Read the model definition and answer for the solid it produces. Units are mm, in the model's axes. A direction names the side the tool comes from. Give positions to 0.01 mm unless a question says otherwise; leave off trailing zeros. Order: outer loops, then holes, each group sorted by start corner. A loop starts at its lowest first (then second) coordinate and runs counter-clockwise, first axis right, second up. Notation, with made-up numbers: (49.25, 45) - (72.25, 45) arc R15 cw to (72.25, 69) - close; hole circle Ø3 at (52.25, 60). An arc over 180 degrees is marked (long way). Use a Markdown table: item, result. Add a question column.
1. Flat-ended cylindrical pins translate along their axes: P1, Ø5, axis at y = -18.5, z = 10, coming from the -X side; P2, Ø12, axis at y = -17.5, z = 13, coming from the -X side; P3, Ø8, axis at x = 19, z = 3, coming from the -Y side. Find the tip coordinate at first contact, or state that the pin passes through.
2. A cutting plane is placed at B-B on x = 0. Determine the outline of the cut face in (y, z).
3. For a pull along Y with two mould halves and no side action, classify faces 1 (the flat face through (14, -14, 0)), 2 (the cylindrical face through (-20.514, 13.631, 9.86)), 3 (the cylindrical face through (-6.94, -31.24, 9.86)) as released by +Y, released by -Y, zero draft, split by the parting line, or undercut.
4. Which of the six approach directions +Z, -Z, +X, -X, +Y, -Y give full straight-line access (tool end or side, diameter ignored) to faces 4 (the flat face through (14, -14, 20)), 5 (the flat face through (-19, -15, 10))?
5. Consider L1, parallel to Y at x = 0, z = 15; L2, parallel to Y at x = 23.5, z = 17.25; L3, parallel to X at y = -13.5, z = 2.75. Determine where each line is inside the solid, lowest interval first.
6. A cutting plane is placed at D-D on y = 13. Determine the outline of the cut face in (x, z).
7. A cutting plane is placed at C-C on z = 7.25. Determine the outline of the cut face in (x, y), and give its area (3 significant figures).
8. A cutting plane is placed at A-A on y = 0. Determine the outline of the cut face in (x, z).
```python
from build123d import *

# Parameters (mm, degrees)
SKETCH_R     = 32
SKETCH_R_2   = 2.1
SKETCH_R_3   = 3
SKETCH_R_4   = 17.5
PAD_DEPTH    = 20
SKETCH001_R  = 5.5
POCKET_DEPTH = 10


with BuildPart() as part:
    # Sketch → Pad (new body)
    with BuildSketch(Plane.XY):
        Circle(SKETCH_R)
        with Locations((0, -26)):
            Circle(SKETCH_R_2, mode=Mode.SUBTRACT)
        with Locations((-22.51666, 13)):
            Circle(SKETCH_R_2, mode=Mode.SUBTRACT)
        with Locations((22.51666, 13)):
            Circle(SKETCH_R_2, mode=Mode.SUBTRACT)
        with Locations((0, 25)):
            Circle(SKETCH_R_3, mode=Mode.SUBTRACT)
        with Locations((-21.650635, -12.5)):
            Circle(SKETCH_R_3, mode=Mode.SUBTRACT)
        with Locations((21.650635, -12.5)):
            Circle(SKETCH_R_3, mode=Mode.SUBTRACT)
        Circle(SKETCH_R_4, mode=Mode.SUBTRACT)
    extrude(amount=PAD_DEPTH)

    # Sketch001 (on Face10 of Pad) → Pocket (cut)
    with BuildSketch(Plane.XY.offset(20)):
        with Locations((0, 25)):
            Circle(SKETCH001_R)
        with Locations((-21.650635, -12.5)):
            Circle(SKETCH001_R)
        with Locations((21.650635, -12.5)):
            Circle(SKETCH001_R)
    extrude(amount=-POCKET_DEPTH, mode=Mode.SUBTRACT)


solid = part.part
```
Output values:
| question | item | result |
|---|---|---|
| 1 | P1 | x = -27.71 |
| 1 | P2 | x = -29.86 |
| 1 | P3 | y = -28.27 |
| 2 | outline | (-32, 0) - (-28.1, 0) - (-28.1, 20) - (-32, 20) - close; (-23.9, 0) - (-17.5, 0) - (-17.5, 20) - (-23.9, 20) - close; (17.5, 0) - (22, 0) - (22, 10) - (19.5, 10) - (19.5, 20) - (17.5, 20) - close; (28, 0) - (32, 0) - (32, 20) - (30.5, 20) - (30.5, 10) - (28, 10) - close |
| 3 | face 1 | zero draft |
| 3 | face 2 | undercut |
| 3 | face 3 | split by the parting line |
| 4 | face 4 | +Z, +X, -X, +Y, -Y |
| 4 | face 5 | +Z |
| 5 | L1 | -32 to -28.1, -23.9 to -17.5, 17.5 to 19.5, 30.5 to 32 |
| 5 | L2 | -21.72 to -17.68, -7.32 to 11.14, 14.86 to 21.72 |
| 5 | L3 | -29.01 to -24.48, -18.82 to -11.14, 11.14 to 18.82, 24.48 to 29.01 |
| 6 | outline | (-29.24, 0) - (-24.62, 0) - (-24.62, 20) - (-29.24, 20) - close; (-20.42, 0) - (-11.72, 0) - (-11.72, 20) - (-20.42, 20) - close; (11.72, 0) - (20.42, 0) - (20.42, 20) - (11.72, 20) - close; (24.62, 0) - (29.24, 0) - (29.24, 20) - (24.62, 20) - close |
| 7 | outline | circle Ø64 at (0, 0); hole circle Ø6 at (-21.65, -12.5); hole circle Ø4.2 at (-22.52, 13); hole circle Ø35 at (0, 0); hole circle Ø6 at (0, 25); hole circle Ø4.2 at (0, -26); hole circle Ø6 at (21.65, -12.5); hole circle Ø4.2 at (22.52, 13) |
| 7 | area | 2,130 mm² |
| 8 | outline | (-32, 0) - (-17.5, 0) - (-17.5, 20) - (-32, 20) - close; (17.5, 0) - (32, 0) - (32, 20) - (17.5, 20) - close |
